Can you work these out from the model? Positions are in its coordinate system, mm. Give positions to 0.01 mm unless a question says otherwise; leave off trailing zeros. Order: outer loops, then holes, each group sorted by start corner. A loop starts at its lowest first (then second) coordinate and runs counter-clockwise, first axis right, second up. Notation, with made-up numbers: (-22.75, 17) - (0.25, 17) arc R31 ccw to (0.25, 48) - close; hole circle Ø11 at (37, 18). An arc over 180 degrees is marked (long way). One line per question, with ' | ' between items.
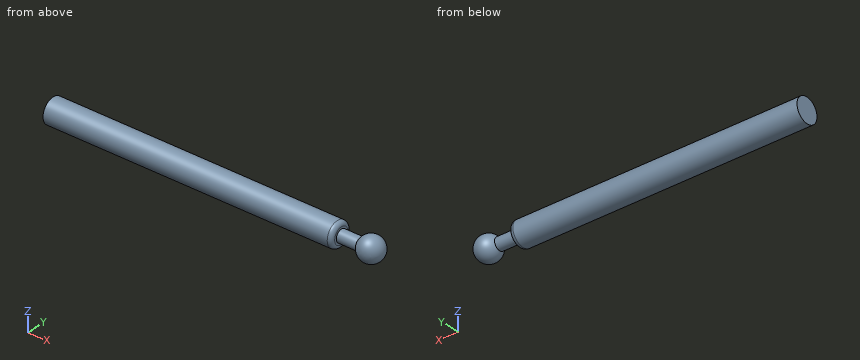
```python
from build123d import *

# Parameters (mm, degrees)
SKETCH2_R           = 3
BOSS_EXTRUDE1_DEPTH = 70
SKETCH3_R           = 1.5
BOSS_EXTRUDE2_DEPTH = 5
FILLET1_R           = 1


with BuildPart() as part:
    # Sketch2 → Boss-Extrude1 (new body)
    with BuildSketch(Plane(origin=(0, 0, 0), x_dir=(0, 0, -1), z_dir=(1, 0, 0))):
        Circle(SKETCH2_R)
    extrude(amount=BOSS_EXTRUDE1_DEPTH)

    # Sketch3 → Boss-Extrude2 (add)
    with BuildSketch(Plane(origin=(70, 0, 0), x_dir=(0, 0, -1), z_dir=(1, 0, 0))):
        Circle(SKETCH3_R)
    extrude(amount=BOSS_EXTRUDE2_DEPTH)

    # Fillet1
    fillet1_edges = [part.edges().sort_by_distance(p)[0] for p in [
        (70, 0, 3),
    ]]
    fillet(fillet1_edges, radius=FILLET1_R)

    # Sketch4 → Revolve1 (revolve)
    with BuildSketch(Plane.XY):
        with BuildLine():
            Line((75, 0), (77.25, 0))
            Line((77.25, 0), (80.25, 0))
            ThreePointArc((80.25, 0), (77.25, -3), (74.25, 0))
            Line((74.25, 0), (75, 0))
        make_face()
    revolve(axis=Axis((75, 0, 0), (1, 0, 0)))


solid = part.part
```
(1) Imagine slicing it at C-C (x = 19). List the corners of the cut face in (y, z) for me.
Answer below:
outline: circle Ø6 at (0, 0)
(2) Imagine slicing it at D-D (x = 75.5). List the corners of the cut face in (y, z) for me.
Answer below:
outline: circle Ø4.87 at (0, 0)
(3) If I drill on line 1 (Z direction, x = 30, y = -0.25); line 2 (X direction, y = -0.75, z = -1.8); line 3 (Y direction, x = 31.5, z = -0.1), over which ranges is the centre line in solid material (lowest first)?
Answer below:
line 1: -2.99 to 2.99 | line 2: 0 to 70, 74.97 to 79.53 | line 3: -3 to 3
(4) Imagine slicing it at A-A (z = 0). List the corners of the cut face in (x, y) for me.
Answer below:
outline: (0, -3) - (69, -3) arc R1 ccw to (70, -2) - (70, -1.5) - (74.65, -1.5) arc R3 ccw (long way) to (74.65, 1.5) - (70, 1.5) - (70, 2) arc R1 ccw to (69, 3) - (0, 3) - close
(5) Will these pins go through, and if not, where does the flat tip stop? pin 1 (2 mm diameter, centred on y = 2, z = 0, fed in from +X); pin 2 (2 mm diameter, centred on x = 15.5, z = -2.5, fed in from -Y); pin 3 (2 mm diameter, centred on x = 38.5, y = 1.5, fed in from +Z).
Answer below:
pin 1: x = 80.08 | pin 2: y = -2.6 | pin 3: z = 2.96
